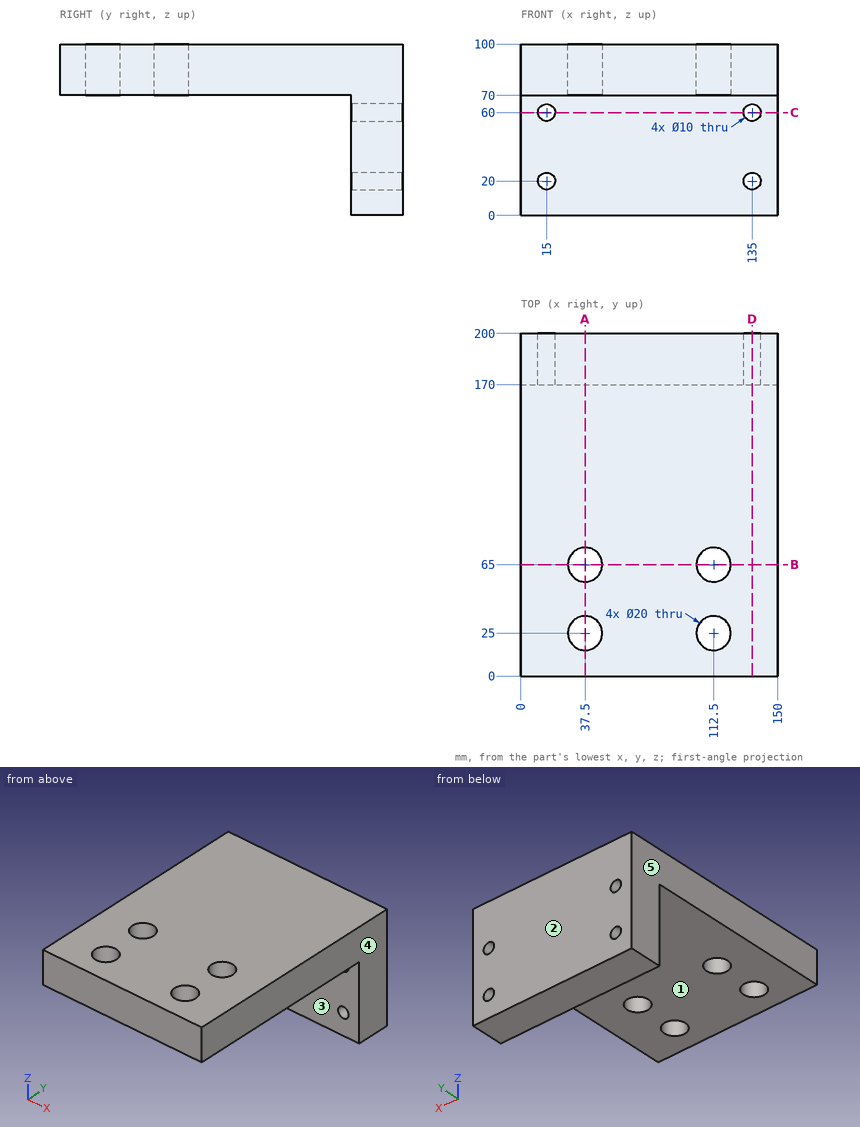
Answer from the drawing. Dimensions are ordinates in mm from the lowest x, y and z of the part. A direction names the side the tool comes from. Give positions to 0.01 mm unless a question says otherwise; leave off trailing zeros. Write each loop counter-clockwise with the first axis right and the second up, starting at its lowest first coordinate (ties: lowest second). Pieces come first, ordered by that corner, then holes.
1) Given P1, Ø13, axis at x = 135, z = 20, coming from the -Y side; P2, Ø8, axis at x = 15, z = 60, coming from the -Y side; P3, Ø5, axis at x = 131, y = 72.5, coming from the -Z side, each flat-ended and moving along its own axis, determine where each tip first touches the part or whether it passes through.
2) Section B-B (y = 65) is taken. Write down the section's boundary in (x, z).
3) Section A-A (x = 37.5) is taken. Write down the section's boundary in (y, z), and give its area (3 significant figures).
4) Find the intervals of material crossed by L1, parallel to X at y = 190, z = 60; L2, parallel to Y at x = 112.5, z = 93.25; L3, parallel to Y at x = 56, z = 26.5, in increasing order.
5) A tool of negligible diameter and unlimited length cuts with its end or side. For the marked faces 1 and 2, from which of +Z, -Z, +X, -X, +Y, -Y can it reach the whole face along a straight path? Write none if from no direction.
6) For a pull along X with two mould halves and no side action, classify the marked faces 3, 4 and 5 as pulls with the +X half, pulls with the -X half, needs draft (parallel to the pull), parting line crosses it, or undercut.
7) Section D-D (x = 135) is taken. Write down the section's boundary in (y, z), and give its area (3 significant figures).
8) Section C-C (z = 60) is taken. Write down the section's boundary in (x, y), and give its area (3 significant figures).
Response:
1. P1: stops at y = 170
1. P2: passes through
1. P3: stops at z = 70
2. outline: (0, 70) - (27.5, 70) - (27.5, 100) - (0, 100) - close; (47.5, 70) - (102.5, 70) - (102.5, 100) - (47.5, 100) - close; (122.5, 70) - (150, 70) - (150, 100) - (122.5, 100) - close
3. outline: (0, 70) - (15, 70) - (15, 100) - (0, 100) - close; (35, 70) - (55, 70) - (55, 100) - (35, 100) - close; (75, 70) - (170, 70) - (170, 0) - (200, 0) - (200, 100) - (75, 100) - close
3. area: 6,900 mm2
4. L1: x = 0 to 10, 20 to 130, 140 to 150
4. L2: y = 0 to 15, 35 to 55, 75 to 200
4. L3: y = 170 to 200
5. face 1: -Z, +X, -X, -Y
5. face 2: +Z, -Z, +X, -X, +Y
6. face 3: needs draft
6. face 4: pulls with the +X half
6. face 5: pulls with the -X half
7. outline: (0, 70) - (170, 70) - (170, 65) - (200, 65) - (200, 100) - (0, 100) - close; (170, 0) - (200, 0) - (200, 15) - (170, 15) - close; (170, 25) - (200, 25) - (200, 55) - (170, 55) - close
7. area: 7,500 mm2
8. outline: (0, 170) - (10, 170) - (10, 200) - (0, 200) - close; (20, 170) - (130, 170) - (130, 200) - (20, 200) - close; (140, 170) - (150, 170) - (150, 200) - (140, 200) - close
8. area: 3,900 mm2
